For this review, take the finished solid that the model builds, in its own axes (mm). A direction names the side the tool comes from. Round coordinates to 2 decimals unless told otherwise and drop trailing zeros. Write each loop counter-clockwise with the first axis right and the second up, starting at its lowest first coordinate (ties: lowest second). Pieces come first, ordered by that corner, then holes. Notation, with made-up numbers: M 13,43.5 L 70,43.5 A11 cw 70,51.5 Z; hole C -35.75,-32.5 d4. An arc over 180 degrees is marked long. Answer in a Markdown table with one row per item.
```python
from build123d import *

# Parameters (mm, degrees)
SKETCH_W        = 93
SKETCH_H        = 59
PAD_DEPTH       = 18
POCKET_DEPTH    = 16
POCKET001_DEPTH = 6
SKETCH003_W     = 25
SKETCH003_H     = 8
POCKET002_DEPTH = 5
SKETCH004_R     = 2.5
SKETCH004_W     = 2
SKETCH004_H     = 20.5
PAD001_DEPTH    = 3
SKETCH005_W     = 23
SKETCH005_H     = 2
PAD002_DEPTH    = 8
SKETCH006_W     = 2
SKETCH006_H     = 2
PAD003_DEPTH    = 2
SKETCH007_R     = 1
POCKET003_DEPTH = 4
POCKET004_DEPTH = 2
POCKET005_DEPTH = 2
SKETCH010_R     = 1
POCKET006_DEPTH = 8
SKETCH011_W     = 10
SKETCH011_H     = 4
POCKET007_DEPTH = 7
FILLET_R        = 2
FILLET001_R     = 4
FILLET002_R     = 3
FILLET003_R     = 1


with BuildPart() as part:
    # Sketch → Pad (new body)
    with BuildSketch(Plane.XY):
        with Locations((46.5, 29.5)):
            Rectangle(SKETCH_W, SKETCH_H)
    extrude(amount=PAD_DEPTH)

    # Sketch001 (on Face6 of Pad) → Pocket (cut)
    with BuildSketch(Plane.XY.offset(18)):
        Polygon((7, 57), (86, 57), (86, 52), (91, 52), (91, 27), (86, 27), (86, 2), (7, 2), (7, 27), (2, 27), (2, 52), (7, 52), align=None)
    extrude(amount=-POCKET_DEPTH, mode=Mode.SUBTRACT)

    # Sketch002 (on Face5 of Pocket) → Pocket001 (cut)
    with BuildSketch(Plane.XY.offset(18)):
        Polygon((0, 20.5), (3, 20.5), (3, 27), (4, 27), (4, 22.75), (7, 22.75), (7, 11.25), (4, 11.25), (4, 7), (3, 7), (3, 13.5), (0, 13.5), align=None)
    extrude(amount=-POCKET001_DEPTH, mode=Mode.SUBTRACT)

    # Sketch003 (on Face14 of Pocket001) → Pocket002 (cut)
    with BuildSketch(Plane.YZ.offset(7)):
        with Locations((14.5, 6)):
            Rectangle(SKETCH003_W, SKETCH003_H)
    extrude(amount=-POCKET002_DEPTH, mode=Mode.SUBTRACT)

    # Sketch004 (on Face31 of Pocket002) → Pad001 (join)
    with BuildSketch(Plane.XY.offset(2)):
        with Locations((23.5, 53.5)):
            Circle(SKETCH004_R)
        with Locations((35.5, 53.5)):
            Circle(SKETCH004_R)
        with Locations((53.5, 53.5)):
            Circle(SKETCH004_R)
        with Locations((53.5, 37)):
            Circle(SKETCH004_R)
        with Locations((35.5, 37)):
            Circle(SKETCH004_R)
        with Locations((65.5, 53.5)):
            Circle(SKETCH004_R)
        with Locations((83.5, 53.5)):
            Circle(SKETCH004_R)
        with Locations((83.5, 37)):
            Circle(SKETCH004_R)
        with Locations((65.5, 37)):
            Circle(SKETCH004_R)
        with Locations((9.5, 53.5)):
            Circle(SKETCH004_R)
        with Locations((24, 12.25)):
            Rectangle(SKETCH004_W, SKETCH004_H)
    extrude(amount=PAD001_DEPTH)

    # Sketch005 (on Face33 of Pad001) → Pad002 (join)
    with BuildSketch(Plane.XY.offset(2)):
        with Locations((13.5, 23.5)):
            Rectangle(SKETCH005_W, SKETCH005_H)
    extrude(amount=PAD002_DEPTH)

    # Sketch006 (on Face30 of Pad002) → Pad003 (join)
    with BuildSketch(Plane.XY.offset(5)):
        with Locations((24, 3)):
            Rectangle(SKETCH006_W, SKETCH006_H)
    extrude(amount=PAD003_DEPTH)

    # Sketch007 (on Face37 of Pad003) → Pocket003 (cut)
    with BuildSketch(Plane.XY.offset(5)):
        with Locations((23.5, 53.5)):
            Circle(SKETCH007_R)
        with Locations((35.5, 53.5)):
            Circle(SKETCH007_R)
        with Locations((9.5, 53.5)):
            Circle(SKETCH007_R)
        with Locations((53.5, 53.5)):
            Circle(SKETCH007_R)
        with Locations((65.5, 53.5)):
            Circle(SKETCH007_R)
        with Locations((83.5, 53.5)):
            Circle(SKETCH007_R)
        with Locations((35.5, 37)):
            Circle(SKETCH007_R)
        with Locations((53.5, 37)):
            Circle(SKETCH007_R)
        with Locations((65.5, 37)):
            Circle(SKETCH007_R)
        with Locations((83.5, 37)):
            Circle(SKETCH007_R)
    extrude(amount=-POCKET003_DEPTH, mode=Mode.SUBTRACT)

    # Sketch008 (on Face49 of Pocket003) → Pocket004 (cut)
    with BuildSketch(Plane(origin=(0, 59, 0), x_dir=(-1, 0, 0), z_dir=(0, 1, 0))):
        with BuildLine():
            ThreePointArc((-79, 6.5), (-76.5, 4), (-74, 6.5))
            Line((-74, 6.5), (-74, 14.5))
            ThreePointArc((-74, 14.5), (-76.5, 17), (-79, 14.5))
            Line((-79, 6.5), (-79, 14.5))
        make_face()
        with BuildLine():
            ThreePointArc((-72, 6.5), (-69.5, 4), (-67, 6.5))
            Line((-67, 6.5), (-67, 14.5))
            ThreePointArc((-67, 14.5), (-69.5, 17), (-72, 14.5))
            Line((-72, 6.5), (-72, 14.5))
        make_face()
        with BuildLine():
            ThreePointArc((-65, 6.5), (-62.5, 4), (-60, 6.5))
            Line((-60, 6.5), (-60, 14.5))
            ThreePointArc((-60, 14.5), (-62.5, 17), (-65, 14.5))
            Line((-65, 6.5), (-65, 14.5))
        make_face()
        with BuildLine():
            ThreePointArc((-58, 6.5), (-55.5, 4), (-53, 6.5))
            Line((-53, 6.5), (-53, 14.5))
            ThreePointArc((-53, 14.5), (-55.5, 17), (-58, 14.5))
            Line((-58, 6.5), (-58, 14.5))
        make_face()
        with BuildLine():
            ThreePointArc((-51, 6.5), (-48.5, 4), (-46, 6.5))
            Line((-46, 6.5), (-46, 14.5))
            ThreePointArc((-46, 14.5), (-48.5, 17), (-51, 14.5))
            Line((-51, 6.5), (-51, 14.5))
        make_face()
        with BuildLine():
            ThreePointArc((-44, 6.5), (-41.5, 4), (-39, 6.5))
            Line((-39, 6.5), (-39, 14.5))
            ThreePointArc((-39, 14.5), (-41.5, 17), (-44, 14.5))
            Line((-44, 6.5), (-44, 14.5))
        make_face()
        with BuildLine():
            ThreePointArc((-37, 6.5), (-34.5, 4), (-32, 6.5))
            Line((-32, 6.5), (-32, 14.5))
            ThreePointArc((-32, 14.5), (-34.5, 17), (-37, 14.5))
            Line((-37, 6.5), (-37, 14.5))
        make_face()
        with BuildLine():
            ThreePointArc((-86, 6.5), (-83.5, 4), (-81, 6.5))
            Line((-81, 6.5), (-81, 14.5))
            ThreePointArc((-81, 14.5), (-83.5, 17), (-86, 14.5))
            Line((-86, 6.5), (-86, 14.5))
        make_face()
    extrude(amount=-POCKET004_DEPTH, mode=Mode.SUBTRACT)

    # Sketch009 (on Face80 of Pocket004) → Pocket005 (cut)
    with BuildSketch(Plane.YZ.offset(93)):
        with BuildLine():
            ThreePointArc((40, 6.5), (42.5, 4), (45, 6.5))
            Line((45, 6.5), (45, 14.5))
            ThreePointArc((45, 14.5), (42.5, 17), (40, 14.5))
            Line((40, 6.5), (40, 14.5))
        make_face()
        with BuildLine():
            ThreePointArc((33, 6.5), (35.5, 4), (38, 6.5))
            Line((38, 6.5), (38, 14.5))
            ThreePointArc((38, 14.5), (35.5, 17), (33, 14.5))
            Line((33, 6.5), (33, 14.5))
        make_face()
        with BuildLine():
            ThreePointArc((47, 6.5), (49.5, 4), (52, 6.5))
            Line((52, 6.5), (52, 14.5))
            ThreePointArc((52, 14.5), (49.5, 17), (47, 14.5))
            Line((47, 6.5), (47, 14.5))
        make_face()
    extrude(amount=-POCKET005_DEPTH, mode=Mode.SUBTRACT)

    # Sketch010 (on Face26 of Pocket005) → Pocket006 (cut)
    with BuildSketch(Plane.XY.offset(18)):
        with Locations((4, 55)):
            Circle(SKETCH010_R)
        with Locations((4, 4)):
            Circle(SKETCH010_R)
        with Locations((89, 4)):
            Circle(SKETCH010_R)
        with Locations((89, 55)):
            Circle(SKETCH010_R)
    extrude(amount=-POCKET006_DEPTH, mode=Mode.SUBTRACT)

    # Sketch011 (on Face93 of Pocket006) → Pocket007 (cut)
    with BuildSketch(Plane(origin=(0, 0, 0), x_dir=(0, -1, 0), z_dir=(-1, 0, 0))):
        with Locations((-12.25, 8.5)):
            Rectangle(SKETCH011_W, SKETCH011_H)
    extrude(amount=-POCKET007_DEPTH, mode=Mode.SUBTRACT)

    # Fillet
    fillet_edges = [part.edges().sort_by_distance(p)[0] for p in [
        (0, 0, 9),
        (93, 0, 9),
    ]]
    fillet(fillet_edges, radius=FILLET_R)

    # Fillet001
    fillet001_edges = [part.edges().sort_by_distance(p)[0] for p in [
        (93, 59, 9),
        (0, 59, 9),
    ]]
    fillet(fillet001_edges, radius=FILLET001_R)

    # Fillet002
    fillet002_edges = [part.edges().sort_by_distance(p)[0] for p in [
        (7, 52, 10),
        (86, 52, 10),
    ]]
    fillet(fillet002_edges, radius=FILLET002_R)

    # Fillet003
    fillet003_edges = [part.edges().sort_by_distance(p)[0] for p in [
        (1, 7.25, 6.5),
        (1, 17.25, 6.5),
        (3.5, 17.25, 10.5),
        (3.5, 7.25, 10.5),
    ]]
    fillet(fillet003_edges, radius=FILLET003_R)


solid = part.part
```
Q1. Insertion check: P1, Ø1.6, axis at x = 24, y = 53, coming from the +Z side; P2, Ø0.6, axis at y = 58.5, z = 10, coming from the -X side; P3, Ø6, axis at x = 30, y = 43, coming from the +Z side. Each pin has a flat end and moves straight along its axis. Give the tip position at first contact, or say it passes through.
Found:
| item | result |
|---|---|
| P1 | z = 5 |
| P2 | x = 1.6 |
| P3 | z = 2 |
Q2. Machinability: for faces 4 (the face through (92, 42.6, 17)), 5 (the face through (5, 20, 10)), 6 (the face through (76.4, 58, 17)), 7 (the face through (2, 13.5, 15)), 8 (the face through (55, 37, 5)), which of the approach directions +Z, -Z, +X, -X, +Y, -Y give a long, thin tool a straight path to every point of the face, cutting with its end or side? Answer none if there is none.
Found:
| item | result |
|---|---|
| face 4 | +X |
| face 5 | none |
| face 6 | +Y |
| face 7 | +Z, -X |
| face 8 | +Z |
Q3. Take a section at C-C (z = 13). State how many separate pieces and enclosed holes the cut face has, then the cut area to 3 significant figures.
Found:
| item | result |
|---|---|
| separate pieces | 13 |
| enclosed holes | 4 |
| area | 681 mm² |
Q4. Take a section at A-A (y = 42.5). State the section outline as (x, z) points, then the cut area to 3 significant figures.
Found:
| item | result |
|---|---|
| outline | M 0,0 L 93,0 L 93,4 L 91,4 L 91,2 L 2,2 L 2,18 L 0,18 Z; M 91,17 L 93,17 L 93,18 L 91,18 Z |
| area | 224 mm² |
Q5. For probe 1 along X at (y, z) = (12, 3.75); probe 2 along X at (y, z) = (31.5, 2.25); probe 3 along X at (y, z) = (25.5, 6), list the stretches that pass through material, from the lowest coordinate up.
Found:
| item | result |
|---|---|
| probe 1 | 0 to 2, 23 to 25, 86 to 93 |
| probe 2 | 0 to 2, 91 to 93 |
| probe 3 | 0 to 2, 86 to 93 |
Q6. Mouldability with a two-part tool opening along Z and no side actions: class faces 1 (the face through (16, 24, 10)), 2 (the face through (1, 12, 6.5)), 3 (the face through (92.4, 0.57, 9.13)) as +Z half, -Z half, draft (parallel to the pull), parting line (faces both ways), or undercut.
Found:
| item | result |
|---|---|
| face 1 | +Z half |
| face 2 | undercut |
| face 3 | draft |
Q7. Take a section at D-D (y = 26). State the section outline as (x, z) points.
Found:
| item | result |
|---|---|
| outline | M 0,0 L 93,0 L 93,18 L 86,18 L 86,2 L 2,2 L 2,10 L 7,10 L 7,18 L 4,18 L 4,12 L 3,12 L 3,18 L 0,18 Z |
Q8. Take a section at B-B (x = 69.5). State the section outline as (y, z) points, then the cut area to 3 significant figures.
Found:
| item | result |
|---|---|
| outline | M 0,0 L 59,0 L 59,4 L 57,4 L 57,2 L 2,2 L 2,18 L 0,18 Z; M 57,17 L 59,17 L 59,18 L 57,18 Z |
| area | 156 mm² |
